from build123d import *

# Parameters (mm, degrees)
SKETCH1_W           = 48
SKETCH1_H           = 5
BOSS_EXTRUDE1_DEPTH = 70


with BuildPart() as part:
    # Sketch1 → Boss-Extrude1 (new body)
    with BuildSketch(Plane.XY):
        Polygon((4, 0), (0, 0), (0, 70), (56, 70), (56, 0), (52, 0), (52, 63), (4, 63), align=None)
        with Locations((28, 32.5)):
            Rectangle(SKETCH1_W, SKETCH1_H)
    extrude(amount=BOSS_EXTRUDE1_DEPTH)


solid = part.part
Build history of the part. All positions in model axes, mm. A direction names the side the tool comes from. Round coordinates to 2 decimals unless told otherwise and drop trailing zeros. Loops run counter-clockwise (first coordinate to the right, second up) from the corner with the lowest first, then second, coordinate; pieces in that order, holes last. Notation, with made-up numbers: (49.25, 81.5) -> (62.25, 81.5) arc R38 cw to (62.25, 119.5) -> close; hole circle Ø10 at (83.5, 4.25). An arc over 180 degrees is marked (long way). Use CSV: the item, a comma, the result in double quotes. Start each with the question number.
Q1. Drill centre lines: L1, parallel to Y at x = 45.5, z = 15; L2, parallel to X at y = 17.5, z = 63. Where is each one in solid material? Low to high.
Q2. Saw through at C-C on z = 30.5. Give the cut face in (x, y).
Q3. Saw through at B-B on y = 36. Give the cut face in (x, z), and give its area (3 significant figures).
Q4. Which spindle directions (+Z, -Z, +X, -X, +Y, -Y) get a long thin tool onto all of the face, cutting with end or side? Do faces 1 (the face through (56, 35, 35)), 2 (the face through (4, 49, 35)), 3 (the face through (52, 15, 35)). Say none if no direction does.
Q5. Saw through at A-A on x = 22. Give the cut face in (y, z).
Q6. Mould opens along Y. For faces 4 (the face through (52, 49, 35)), 5 (the face through (28, 30, 35)), 6 (the face through (28, 33, 70)) say: +Y half, -Y half, draft (parallel to the pull), parting line (faces both ways), or undercut.
Q7. Flat gauge pin, fed straight in: pin 1 Ø1.5 at (x, z) = (27, 15) entering from -Y. Where does the tip first touch, or does it go through?
Solutions:
1,L1,"y = 30 to 35, 63 to 70"
1,L2,"x = 0 to 4, 52 to 56"
2,outline,"(0, 0) -> (4, 0) -> (4, 30) -> (52, 30) -> (52, 0) -> (56, 0) -> (56, 70) -> (0, 70) -> close; hole (4, 35) -> (52, 35) -> (52, 63) -> (4, 63) -> close"
3,outline,"(0, 0) -> (4, 0) -> (4, 70) -> (0, 70) -> close; (52, 0) -> (56, 0) -> (56, 70) -> (52, 70) -> close"
3,area,"560 mm^2"
4,face 1,"+Z, -Z, +X, +Y, -Y"
4,face 2,"+Z, -Z"
4,face 3,"+Z, -Z, -Y"
5,outline,"(30, 0) -> (35, 0) -> (35, 70) -> (30, 70) -> close; (63, 0) -> (70, 0) -> (70, 70) -> (63, 70) -> close"
6,face 4,"undercut"
6,face 5,"-Y half"
6,face 6,"draft"
7,pin 1,"stops at y = 30"
